```python
from build123d import *

# Parameters (mm, degrees)
PAD_DEPTH    = 3
POCKET_DEPTH = 3.001


with BuildPart() as part:
    # Sketch → Pad (new body)
    with BuildSketch(Plane.XZ):
        with BuildLine():
            ThreePointArc((6, 40), (1.757359, 38.242641), (0, 34))
            Line((0, 6), (0, 34))
            ThreePointArc((0, 6), (1.757359, 1.757359), (6, 0))
            Line((144, 0), (6, 0))
            ThreePointArc((144, 0), (148.242641, 1.757359), (150, 6))
            Line((150, 34), (150, 6))
            ThreePointArc((150, 34), (148.242641, 38.242641), (144, 40))
            Line((6, 40), (144, 40))
        make_face()
    extrude(amount=PAD_DEPTH)

    # Sketch001 (on Face9 of Pad) → Pocket (cut, through all)
    with BuildSketch(Plane(origin=(0, 0, 0), x_dir=(1, 0, 0), z_dir=(0, 1, 0))):
        with BuildLine():
            ThreePointArc((45, -30), (43, -32), (45, -34))
            Line((45, -34), (65, -34))
            ThreePointArc((65, -34), (67, -32), (65, -30))
            Line((65, -30), (45, -30))
        make_face()
    extrude(amount=-POCKET_DEPTH, mode=Mode.SUBTRACT)


solid = part.part
```
Design review of the part built by this model. Coordinates are the model's own, in mm. A direction names the side the tool comes from. Coordinates: 2 decimals unless noted, no trailing zeros. Order: outer loops, then holes, each group sorted by start corner. A loop starts at its lowest first (then second) coordinate and runs counter-clockwise, first axis right, second up. Notation, with made-up numbers: M 76.25,57.25 L 93.25,57.25 A27 cw 93.25,77.25 Z; hole C -7,-31 d4. An arc over 180 degrees is marked long. Answer as a JSON object with one key per item and string values. Group by question number.
1) Add section B-B, the plane z = 32. Write out the cut boundary in (x, y), then the cut area to 3 significant figures.
2) Tool access review of faces 1 (the flat face through (76, -1, 0)), 2 (the flat face through (55, -1, 30)): name each direction out of +Z, -Z, +X, -X, +Y, -Y from which nothing blocks a thin tool from reaching the whole face with its end or side.
3) Add section C-C, the plane y = -2.5. Write out the cut boundary in (x, z).
4) Mouldability with a two-part tool opening along Z and no side actions: class faces 3 (the flat face through (150, -1, 20)), 4 (the cylindrical face through (148.289, -1.479, 38.196)), 5 (the cylindrical face through (43, -1, 32)) as pulls with the +Z half, pulls with the -Z half, needs draft (parallel to the pull), parting line crosses it, or undercut.
5) Add section A-A, the plane x = 60. Write out the cut boundary in (y, z), then the cut area to 3 significant figures.
6) Wall thickness on L1, parallel to Z at x = 51, y = -1.75; L2, parallel to X at y = -2.25, z = 33; L3, parallel to X at y = -1.55, z = 32.5: over which ranges is each line inside the solid? List them lowest first.
Computed values:
{
 "1": {"outline": "M 0,-3 L 43,-3 L 43,0 L 0,0 Z; M 67,-3 L 150,-3 L 150,0 L 67,0 Z", "area": "378 mm^2"},
 "2": {"face 1": "-Z, +X, -X, +Y, -Y", "face 2": "+Y, -Y"},
 "3": {"outline": "M 0,6 A6 ccw 6,0 L 144,0 A6 ccw 150,6 L 150,34 A6 ccw 144,40 L 6,40 A6 ccw 0,34 Z; hole M 45,30 L 65,30 A2 ccw 65,34 L 45,34 A2 ccw Z"},
 "4": {"face 3": "needs draft", "face 4": "pulls with the +Z half", "face 5": "undercut"},
 "5": {"outline": "M -3,0 L 0,0 L 0,30 L -3,30 Z; M -3,34 L 0,34 L 0,40 L -3,40 Z", "area": "108 mm^2"},
 "6": {"L1": "z = 0 to 30, 34 to 40", "L2": "x = 0 to 43.27, 66.73 to 150", "L3": "x = 0 to 43.06, 66.94 to 150"}
}
